from build123d import *

# Parameters (mm, degrees)
F1_DEPTH = 50
F3_R     = 150
F4_DEPTH = 10
F3_R_2   = 141.1224
F3_R_3   = 40
F5_DEPTH = 10


with BuildPart() as f1:
    # F0 (on Top) → F1 (new body)
    with BuildSketch(Plane.XY):
        Polygon((160, -92.376043), (160, 92.376043), (0, 184.752086), (-160, 92.376043), (-160, -92.376043), (0, -184.752086), align=None)
    extrude(amount=F1_DEPTH)

    # F3 (on face) → F4 (join)
    with BuildSketch(Plane.XY.offset(50)):
        Polygon((-160, -92.376043), (0, -184.752086), (160, -92.376043), (160, 92.376043), (0, 184.752086), (-160, 92.376043), align=None)
        Circle(F3_R, mode=Mode.SUBTRACT)
    extrude(amount=F4_DEPTH)

    # F3 (on face) → F5 (join)
    with BuildSketch(Plane.XY.offset(50)):
        Circle(F3_R_2)
        Circle(F3_R_3, mode=Mode.SUBTRACT)
    extrude(amount=F5_DEPTH)


solid = f1.part
CAD build for the part. Positions are in the model's coordinates, mm. A direction names the side the tool comes from. Round coordinates to 2 decimals unless told otherwise and drop trailing zeros. Write each loop counter-clockwise with the first axis right and the second up, starting at its lowest first coordinate (ties: lowest second). Pieces come first, ordered by that corner, then holes.
(1) Mould opens along X. For faces 3 (the face through (-8.67, -39.05, 54.93)), 4 (the face through (110.4, -88.2, 50)), 5 (the face through (-78.9, 139.2, 29.6)), 6 (the face through (160, -1, 30)) say: pulls with the +X half, pulls with the -X half, needs draft (parallel to the pull), parting line crosses it, or undercut.
(2) Probe line 1 along Y through (x, z) = (0, 54); line 2 along Y through (x, z) = (114.5, 54.5); line 3 along Z through (x, y) = (-33.5, 11.5). List the from-to ranges inside material, lowest first.
(3) Drop flat-ended pins along their axis: P1, Ø1, axis at x = -6.5, z = 53.5, coming from the +Y side; P2, Ø1.5, axis at x = -37.5, z = 46, coming from the -Y side; P3, Ø24, axis at x = -8.5, y = -11.5, coming from the +Z side. Give the stop position or say it passes through.
(4) Slice it at D-D, the plane y = 115. Write the cut outline in (x, z), and give its area (3 significant figures).
(5) 3-axis set-ups, long thin cutter, end or side, ignore diameter. For faces 1 (the face through (-19.527, 148.724, 54.93)), 2 (the face through (-160, 1, 30)): which of +Z, -Z, +X, -X, +Y, -Y reach the whole face in a straight line?
(6) Slice it at C-C, the plane x = 116. Write the cut outline in (y, z), and give its area (3 significant figures).
(7) Slice it at A-A, the plane y = 0. Write the cut outline in (x, z).
(8) Slice it at B-B, the plane z = 30. Write the cut outline in (x, y), and give its area (3 significant figures).
From the geometry:
1. face 3: undercut
1. face 4: undercut
1. face 5: pulls with the -X half
1. face 6: pulls with the +X half
2. line 1: y = -184.75 to -150, -141.12 to -40, 40 to 141.12, 150 to 184.75
2. line 2: y = -118.65 to -96.9, -82.49 to 82.49, 96.9 to 118.65
2. line 3: z = 0 to 50
3. P1: stops at y = 181.29
3. P2: stops at y = -163.53
3. P3: stops at z = 50
4. outline: (-120.81, 0) - (120.81, 0) - (120.81, 60) - (96.31, 60) - (96.31, 50) - (81.8, 50) - (81.8, 60) - (-81.8, 60) - (-81.8, 50) - (-96.31, 50) - (-96.31, 60) - (-120.81, 60) - close
4. area: 14,200 mm2
5. face 1: +Z
5. face 2: +Z, -Z, -X, +Y, -Y
6. outline: (-117.78, 0) - (117.78, 0) - (117.78, 60) - (95.1, 60) - (95.1, 50) - (80.37, 50) - (80.37, 60) - (-80.37, 60) - (-80.37, 50) - (-95.1, 50) - (-95.1, 60) - (-117.78, 60) - close
6. area: 13,800 mm2
7. outline: (-160, 0) - (160, 0) - (160, 60) - (150, 60) - (150, 50) - (141.12, 50) - (141.12, 60) - (40, 60) - (40, 50) - (-40, 50) - (-40, 60) - (-141.12, 60) - (-141.12, 50) - (-150, 50) - (-150, 60) - (-160, 60) - close
8. outline: (-160, -92.38) - (0, -184.75) - (160, -92.38) - (160, 92.38) - (0, 184.75) - (-160, 92.38) - close
8. area: 88,700 mm2
